Work out the finished part from the listing and answer in its coordinate system (mm). A direction names the side the tool comes from. Round coordinates to 2 decimals unless told otherwise and drop trailing zeros. Order: outer loops, then holes, each group sorted by start corner. A loop starts at its lowest first (then second) coordinate and runs counter-clockwise, first axis right, second up. Notation, with made-up numbers: (86.5, 32) - (121.5, 32) arc R21 cw to (121.5, 71) - close; hole circle Ø7 at (-15.75, 31.25). An arc over 180 degrees is marked (long way). Answer in a Markdown table with one row per item.
from build123d import *

# Parameters (mm, degrees)
F0_R     = 4.258407
F0_R_2   = 4.806756
F0_R_3   = 4.543111
F0_R_4   = 4.869038
F1_DEPTH = 12
F2_DEPTH = 8
F0_R_5   = 24.829414
F3_DEPTH = 7
F0_R_6   = 20.038363
F4_DEPTH = 10


with BuildPart() as f1:
    # F0 (on Front) → F1 (new body)
    with BuildSketch(Plane.XZ):
        with BuildLine():
            Line((61.549276, 45.996532), (-58.450724, 45.996532))
            ThreePointArc((-58.450724, 45.996532), (-62.940852, 44.13666), (-64.800724, 39.646532))
            Line((-64.800724, 39.646532), (-64.800724, -40.353468))
            ThreePointArc((-64.800724, -40.353468), (-62.940852, -44.843596), (-58.450724, -46.703468))
            Line((-58.450724, -46.703468), (61.549276, -46.703468))
            ThreePointArc((61.549276, -46.703468), (66.039404, -44.843596), (67.899276, -40.353468))
            Line((67.899276, -40.353468), (67.899276, 39.646532))
            ThreePointArc((67.899276, 39.646532), (66.039404, 44.13666), (61.549276, 45.996532))
        make_face()
        with Locations((-58.450724, -40.353468)):
            Circle(F0_R, mode=Mode.SUBTRACT)
        with BuildLine():
            ThreePointArc((-54.108147, 30.331052), (-52.248275, 34.82118), (-47.758147, 36.681052))
            Line((-47.758147, 36.681052), (48.495564, 36.681052))
            ThreePointArc((48.495564, 36.681052), (52.985692, 34.82118), (54.845564, 30.331052))
            Line((54.845564, 30.331052), (54.845564, -34.668948))
            ThreePointArc((54.845564, -34.668948), (52.985692, -39.159076), (48.495564, -41.018948))
            Line((48.495564, -41.018948), (-47.758147, -41.018948))
            ThreePointArc((-47.758147, -41.018948), (-52.248275, -39.159076), (-54.108147, -34.668948))
            Line((-54.108147, -34.668948), (-54.108147, 30.331052))
        make_face(mode=Mode.SUBTRACT)
        with Locations((61.549276, -40.353468)):
            Circle(F0_R_2, mode=Mode.SUBTRACT)
        with Locations((-58.450724, 37.651211)):
            Circle(F0_R_3, mode=Mode.SUBTRACT)
        with Locations((61.549276, 39.646532)):
            Circle(F0_R_4, mode=Mode.SUBTRACT)
    extrude(amount=F1_DEPTH)

    # F0 (on Front) → F2 (join)
    with BuildSketch(Plane.XZ):
        with BuildLine():
            Line((48.495564, 36.681052), (-47.758147, 36.681052))
            ThreePointArc((-47.758147, 36.681052), (-52.248275, 34.82118), (-54.108147, 30.331052))
            Line((-54.108147, 30.331052), (-54.108147, -34.668948))
            ThreePointArc((-54.108147, -34.668948), (-52.248275, -39.159076), (-47.758147, -41.018948))
            Line((-47.758147, -41.018948), (48.495564, -41.018948))
            ThreePointArc((48.495564, -41.018948), (52.985692, -39.159076), (54.845564, -34.668948))
            Line((54.845564, -34.668948), (54.845564, 30.331052))
            ThreePointArc((54.845564, 30.331052), (52.985692, 34.82118), (48.495564, 36.681052))
        make_face()
        with BuildLine():
            ThreePointArc((-45.996532, 22.870242), (-44.13666, 27.36037), (-39.646532, 29.220242))
            Line((-39.646532, 29.220242), (40.353468, 29.220242))
            ThreePointArc((40.353468, 29.220242), (44.843596, 27.36037), (46.703468, 22.870242))
            Line((46.703468, 22.870242), (46.703468, -28.216533))
            ThreePointArc((46.703468, -28.216533), (44.843596, -32.706661), (40.353468, -34.566533))
            Line((40.353468, -34.566533), (-39.646532, -34.566533))
            ThreePointArc((-39.646532, -34.566533), (-44.13666, -32.706661), (-45.996532, -28.216533))
            Line((-45.996532, -28.216533), (-45.996532, 22.870242))
        make_face(mode=Mode.SUBTRACT)
    extrude(amount=F2_DEPTH)

    # F0 (on Front) → F3 (join)
    with BuildSketch(Plane.XZ):
        with BuildLine():
            Line((40.353468, 29.220242), (-39.646532, 29.220242))
            ThreePointArc((-39.646532, 29.220242), (-44.13666, 27.36037), (-45.996532, 22.870242))
            Line((-45.996532, 22.870242), (-45.996532, -28.216533))
            ThreePointArc((-45.996532, -28.216533), (-44.13666, -32.706661), (-39.646532, -34.566533))
            Line((-39.646532, -34.566533), (40.353468, -34.566533))
            ThreePointArc((40.353468, -34.566533), (44.843596, -32.706661), (46.703468, -28.216533))
            Line((46.703468, -28.216533), (46.703468, 22.870242))
            ThreePointArc((46.703468, 22.870242), (44.843596, 27.36037), (40.353468, 29.220242))
        make_face()
        Circle(F0_R_5, mode=Mode.SUBTRACT)
    extrude(amount=F3_DEPTH)

    # F0 (on Front) → F4 (join)
    with BuildSketch(Plane.XZ):
        Circle(F0_R_5)
        Circle(F0_R_6, mode=Mode.SUBTRACT)
    extrude(amount=F4_DEPTH)


solid = f1.part
1) Find section C-C, the plane y = -3. Give the vertices of the cut face in (x, z).
Filled in:
| item | result |
|---|---|
| outline | (-64.8, -40.35) arc R6.35 ccw to (-58.45, -46.7) - (61.55, -46.7) arc R6.35 ccw to (67.9, -40.35) - (67.9, 39.65) arc R6.35 ccw to (61.55, 46) - (-58.45, 46) arc R6.35 ccw to (-64.8, 39.65) - close; hole circle Ø9.09 at (-58.45, 37.65); hole circle Ø8.52 at (-58.45, -40.35); hole circle Ø40.08 at (0, 0); hole circle Ø9.74 at (61.55, 39.65); hole circle Ø9.61 at (61.55, -40.35) |
2) The mould has two halves that part along Z. Classify faces 3 (the face through (-64.801, -6, 0)), 4 (the face through (-4.344, -4.93, -19.562)), 5 (the face through (-62.891, -5.916, 44.186)), 6 (the face through (-62.99, -5.916, -44.794)): released by +Z, released by -Z, zero draft, split by the parting line, or undercut.
Filled in:
| item | result |
|---|---|
| face 3 | zero draft |
| face 4 | undercut |
| face 5 | released by +Z |
| face 6 | released by -Z |
3) Find the intervals of material crossed by probe 1 along X at (y, z) = (-9.75, -14.5); probe 2 along Z at (x, y) = (58.5, -5.75); probe 3 along Z at (x, y) = (-46.5, -11.25), in increasing order. Write a range as from..to.
Filled in:
| item | result |
|---|---|
| probe 1 | x = -64.8..-54.11, -20.16..-13.83, 13.83..20.16, 54.85..67.9 |
| probe 2 | z = -46.7..-44.07, -36.64..35.85, 43.44..46 |
| probe 3 | z = -46.7..-41.02, 36.68..46 |
4) Find section D-D, the plane x = -27. Give the vertices of the cut face in (y, z), then the cut area to 3 significant figures.
Filled in:
| item | result |
|---|---|
| outline | (-12, -46.7) - (0, -46.7) - (0, 46) - (-12, 46) - (-12, 36.68) - (-8, 36.68) - (-8, 29.22) - (-7, 29.22) - (-7, -34.57) - (-8, -34.57) - (-8, -41.02) - (-12, -41.02) - close |
| area | 738 mm^2 |
5) Which of the six approach directions +Z, -Z, +X, -X, +Y, -Y give full straight-line access (tool end or side, diameter ignored) to faces 1 (the face through (0, -10, 36.681)), 2 (the face through (-59.37, -5.92, -44.51))?
Filled in:
| item | result |
|---|---|
| face 1 | -Y |
| face 2 | +Y, -Y |
6) This flat-tipped pin is pushed along its axis until it touches: pin 1 (1.5 mm diameter, centred on x = 31.5, z = 10, fed in from -Y). Where does it stop, or does it pass through?
Filled in:
| item | result |
|---|---|
| pin 1 | stops at y = -7 |
7) Find section A-A, the plane x = 0. Give the vertices of the cut face in (y, z), then the cut area to 3 significant figures.
Filled in:
| item | result |
|---|---|
| outline | (-12, -46.7) - (0, -46.7) - (0, -20.04) - (-10, -20.04) - (-10, -24.83) - (-7, -24.83) - (-7, -34.57) - (-8, -34.57) - (-8, -41.02) - (-12, -41.02) - close; (-12, 36.68) - (-8, 36.68) - (-8, 29.22) - (-7, 29.22) - (-7, 24.83) - (-10, 24.83) - (-10, 20.04) - (0, 20.04) - (0, 46) - (-12, 46) - close |
| area | 486 mm^2 |
8) Find section B-B, the plane z = 0. Give the vertices of the cut face in (x, y).
Filled in:
| item | result |
|---|---|
| outline | (-64.8, -12) - (-54.11, -12) - (-54.11, -8) - (-46, -8) - (-46, -7) - (-24.83, -7) - (-24.83, -10) - (-20.04, -10) - (-20.04, 0) - (-64.8, 0) - close; (20.04, -10) - (24.83, -10) - (24.83, -7) - (46.7, -7) - (46.7, -8) - (54.85, -8) - (54.85, -12) - (67.9, -12) - (67.9, 0) - (20.04, 0) - close |
